```python
from build123d import *

# Parameters (mm, degrees)
SKETCH1_R           = 14.3
BOSS_EXTRUDE1_DEPTH = 914.4


with BuildPart() as part:
    # Sketch1 → Boss-Extrude1 (new body)
    with BuildSketch(Plane(origin=(457.2, 0, 0), x_dir=(0, 0, -1), z_dir=(1, 0, 0))):
        with BuildLine():
            Line((-0.25, -15.873031374), (0, -15.575))
            Line((0, -15.575), (0.25, -15.873031374))
            ThreePointArc((0.25, -15.873031374), (11.225320151, -11.225320151), (15.873031374, -0.25))
            Line((15.873031374, -0.25), (15.575, 0))
            Line((15.575, 0), (15.873031374, 0.25))
            ThreePointArc((15.873031374, 0.25), (11.225320151, 11.225320151), (0.25, 15.873031374))
            Line((0.25, 15.873031374), (0, 15.575))
            Line((0, 15.575), (-0.25, 15.873031374))
            ThreePointArc((-0.25, 15.873031374), (-11.225320151, 11.225320151), (-15.873031374, 0.25))
            Line((-15.873031374, 0.25), (-15.575, 0))
            Line((-15.575, 0), (-15.873031374, -0.25))
            ThreePointArc((-15.873031374, -0.25), (-11.225320151, -11.225320151), (-0.25, -15.873031374))
        make_face()
        with Locations(Location((0, 0, 0), (0, 0, 180))):
            Circle(SKETCH1_R, mode=Mode.SUBTRACT)
    extrude(amount=-BOSS_EXTRUDE1_DEPTH)


solid = part.part
```
Can you work these out from the model? Positions are in its coordinate system, mm. Give positions to 0.01 mm unless a question says otherwise; leave off trailing zeros. Loops run counter-clockwise (first coordinate to the right, second up) from the corner with the lowest first, then second, coordinate; pieces in that order, holes last. Notation, with made-up numbers: M -3,-20 L 19,-20 A27 cw 19,10 Z; hole C -5.75,-3.5 d10. An arc over 180 degrees is marked long. Use one line per item in the form item = value. Start each with the question number.
(1) Thinking about a two-plate mould opening in Y: for faces 1 (the cylindrical face through (6.4, 11.35, 11.1)), 2 (the flat face through (457.2, 8.3, 11.83)), 3 (the cylindrical face through (6.4, -14.18, -1.86)), which applies, released by +Y, released by -Y, zero draft, split by the parting line, or undercut?
(2) I want a section at A-A, the plane x = 354. Write out the boundary of the cut face in (y, z) (3 decimals), and give its area (3 significant figures).
(3) Please list where these lines run through material, in increasing order: line 1 (Y direction, x = 213, z = 0) (3 decimals); line 2 (Z direction, x = 285, y = -8); line 3 (Z direction, x = 134, y = 1) (3 decimals).
(4) I want a section at B-B, the plane y = -7.5. Write out the boundary of the cut face in (x, z).
(5) I'm going to push flat-ended pins straight in: P1, Ø6, axis at x = 165.5, z = 11.5, coming from the -Y side; P2, Ø5, axis at x = -154.5, z = 3, coming from the +Y side; P3, Ø1.5, axis at x = 52, y = -12.5, coming from the -Z side. Where does each tip first touch, or does it pass through?
Worked out:
q1.face_1 = released by +Y
q1.face_2 = zero draft
q1.face_3 = undercut
q2.outline = M -15.873,-0.25 A15.875 ccw -0.25,-15.873 L 0,-15.575 L 0.25,-15.873 A15.875 ccw 15.873,-0.25 L 15.575,0 L 15.873,0.25 A15.875 ccw 0.25,15.873 L 0,15.575 L -0.25,15.873 A15.875 ccw -15.873,0.25 L -15.575,0 Z; hole C 0,0 d28.6
q2.area = 149 mm²
q3.line_1 = -15.575 to -14.3, 14.3 to 15.575
q3.line_2 = -13.71 to -11.85, 11.85 to 13.71
q3.line_3 = -15.843 to -14.265, 14.265 to 15.843
q4.outline = M -457.2,-13.99 L 457.2,-13.99 L 457.2,-12.18 L -457.2,-12.18 Z; M -457.2,12.18 L 457.2,12.18 L 457.2,13.99 L -457.2,13.99 Z
q5.P1 = -13.41
q5.P2 = 15.87
q5.P3 = -10.67
